from build123d import *

# Parameters (mm, degrees)
F0_R     = 104.775
F1_DEPTH = 31.75
F2_R     = 58.7375
F3_DEPTH = 14.2875
F3_TAPER = 3
F4_R     = 45.339
F5_DEPTH = 46.0385001
F10_D    = 22.225


with BuildPart() as f1:
    # F0 (on Top) → F1 (new body)
    with BuildSketch(Plane.XY):
        Circle(F0_R)
    extrude(amount=-F1_DEPTH)

    # F2 (on face) → F3 (join)
    with BuildSketch(Plane(origin=(0, 0, -31.75), x_dir=(1, 0, 0), z_dir=(0, 0, -1))):
        Circle(F2_R)
    extrude(amount=F3_DEPTH, taper=F3_TAPER)

    # F4 (on face) → F5 (cut, through all)
    with BuildSketch(Plane.XY):
        Circle(F4_R)
    extrude(amount=-F5_DEPTH, mode=Mode.SUBTRACT)

    # F6 (on Front) → F8 (revolve, cut)
    with BuildSketch(Plane.XZ):
        Polygon((61.9125, -7.9375), (61.9125, 0), (55.959375, 0), (59.3286438537, -7.9375), align=None)
        Polygon((67.865625, 0), (61.9125, 0), (61.9125, -7.9375), (64.4963561463, -7.9375), align=None)
    revolve(axis=Axis((0, 0, 0), (0, 0, 1)), mode=Mode.SUBTRACT)

    # F10 (through all)
    with Locations(Plane.XY):
        with Locations((59.4941968021, 59.4941968021), (84.1375, 0), (59.4941968021, -59.4941968021), (0, -84.1375), (-59.4941968021, -59.4941968021), (-84.1375, 0), (-59.4941968021, 59.4941968021), (0, 84.1375)):
            Hole(F10_D / 2)


solid = f1.part
The listing builds one solid part. Answer for the finished solid, in the listing's coordinates (mm). A direction names the side the tool comes from. Coordinates: 2 decimals unless noted, no trailing zeros. Return JSON: item names as keys, results as strings.
1. Each of these flat-tipped pins is pushed along its axis until it touches: pin 1 Ø1.5 at (x, y) = (-76.5, 55.5) entering from -Z; pin 2 Ø4 at (x, y) = (-67.5, 57.5) entering from -Z; pin 3 Ø6 at (x, z) = (-6.5, -36.5) entering from +Y; pin 4 Ø10 at (y, z) = (-61.5, -6.5) entering from -X. Where does it stop, or does it pass through?
Final values:
{"pin 1": "z = -31.75", "pin 2": "through", "pin 3": "y = 58.44", "pin 4": "x = -88.24"}
2. The part is cut by section A-A on x = 0. Count the separate pieces of the cut face and the enclosed holes in it, then the cut area to 3 significant figures.
Final values:
{"separate pieces": "4", "enclosed holes": "0", "area": "2,600 mm^2"}
3. Consider line 1 along Y through (x, z) = (0, -12) (3 decimals); line 2 along X through (y, z) = (14, -4); line 3 along X through (y, z) = (36, -7.5). Determine where each line is inside the solid, lowest interval first.
Final values:
{"line 1": "-104.775 to -95.25, -73.025 to -45.339, 45.339 to 73.025, 95.25 to 104.775", "line 2": "-103.84 to -64.67, -55.93 to -43.12, 43.12 to 55.93, 64.67 to 103.84", "line 3": "-98.4 to -53.74, -46.92 to -27.56, 27.56 to 46.92, 53.74 to 98.4"}
4. For a pull along X with two mould halves and no side action, classify faces 4 (the face through (0, 46, 0)), 5 (the face through (-22.713, -102.283, -15.653)), 6 (the face through (-5.97, 93.51, -16.1)) as +X half, -X half, draft (parallel to the pull), parting line (faces both ways), or undercut.
Final values:
{"face 4": "draft", "face 5": "parting line", "face 6": "undercut"}
5. Which of the six approach directions +Z, -Z, +X, -X, +Y, -Y give full straight-line access (tool end or side, diameter ignored) to faces 1 (the face through (-28.4, -52.3, -7.938)), 2 (the face through (45, -45, -31.75)), 3 (the face through (-51.3, 67, -16.1))?
Final values:
{"face 1": "+Z", "face 2": "-Z", "face 3": "+Z, -Z"}
